For this review, use the dimensioned drawing (mm, ordinates from the lowest corner) and the shaded views. A direction names the side the tool comes from. Round coordinates to 2 decimals unless told otherwise and drop trailing zeros. Order: outer loops, then holes, each group sorted by start corner. A loop starts at its lowest first (then second) coordinate and runs counter-clockwise, first axis right, second up. Notation, with made-up numbers: M -34.5,48.25 L 16.5,48.25 A31 cw 16.5,84.25 Z; hole C -30,-18.5 d11. An arc over 180 degrees is marked long. One line per item, written item: value. Start each with the question number.
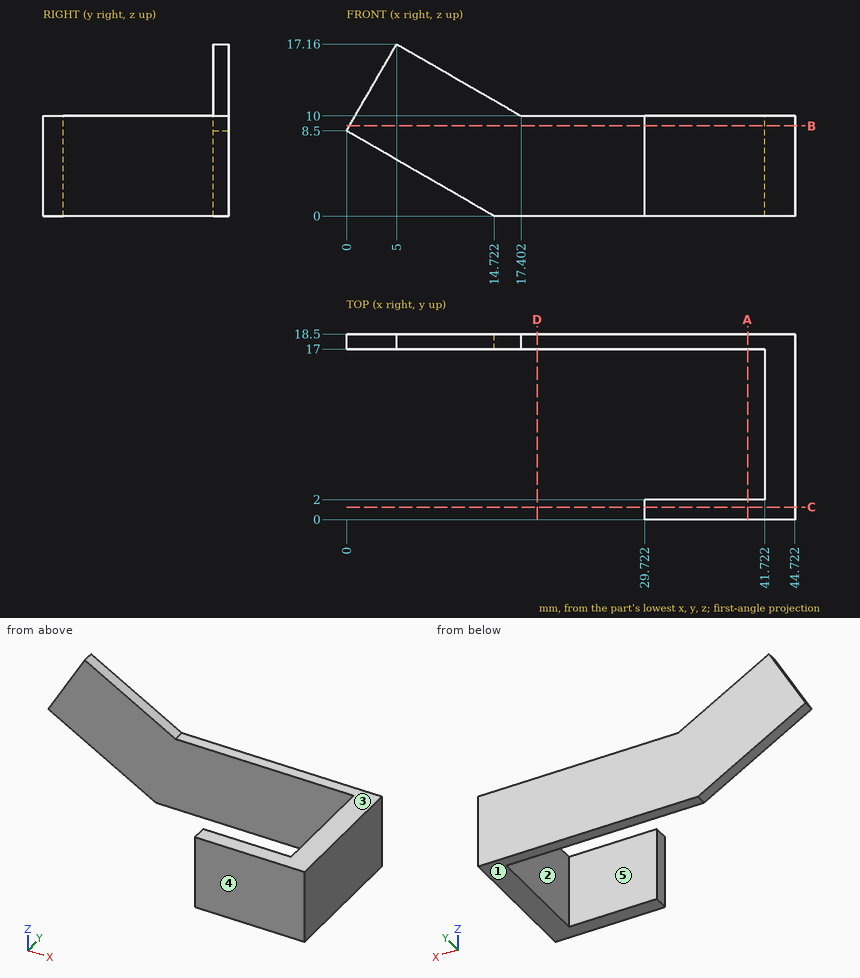
Item 1: Wall thickness on L1, parallel to X at y = 7.25, z = 8; L2, parallel to Y at x = 28.5, z = 6; L3, parallel to Y at x = 33.5, z = 6.25: over which ranges is each line inside the solid? List them lowest first.
Item 2: The part is to be moulded in two halves that separate along Y. For the marked faces 3, 4 and 5, say which applies: pulls with the +Y half, pulls with the -Y half, needs draft (parallel to the pull), parting line crosses it, or undercut.
Item 3: Consider section B-B, the plane z = 9. Give the boundary of the cut face in (x, y).
Item 4: Consider section D-D, the plane x = 19. Give the boundary of the cut face in (y, z).
Item 5: Consider section C-C, the plane y = 1.25. Give the boundary of the cut face in (x, z).
Item 6: Clearance check with flat-ended pins moving along their axes: P1, Ø6, axis at x = 40, y = 3, coming from the -Z side; P2, Ø10, axis at x = 17.5, z = 10.5, coming from the -Y side; P3, Ø1.6, axis at y = 1, z = 7.5, coming from the -X side; P4, Ø4, axis at y = 12.5, z = 13, coming from the -X side. State where each tip first meets the part, or that it passes through.
Item 7: Machinability: for the marked faces 1 and 2, which of the approach directions +Z, -Z, +X, -X, +Y, -Y give a long, thin tool a straight path to every point of the face, cutting with its end or side? Answer none if there is none.
Item 8: Consider section A-A, the plane x = 40. Give the boundary of the cut face in (y, z).
Computed:
1. L1: x = 41.72 to 44.72
1. L2: y = 17 to 18.5
1. L3: y = 0 to 2, 17 to 18.5
2. face 3: needs draft
2. face 4: pulls with the -Y half
2. face 5: undercut
3. outline: M 0.29,17 L 41.72,17 L 41.72,2 L 29.72,2 L 29.72,0 L 44.72,0 L 44.72,18.5 L 0.29,18.5 Z
4. outline: M 17,0 L 18.5,0 L 18.5,10 L 17,10 Z
5. outline: M 29.72,0 L 44.72,0 L 44.72,10 L 29.72,10 Z
6. P1: stops at z = 0
6. P2: stops at y = 17
6. P3: stops at x = 29.72
6. P4: passes through
7. face 1: -Z, +X, -X, +Y, -Y
7. face 2: +Z, -Z, -X
8. outline: M 0,0 L 2,0 L 2,10 L 0,10 Z; M 17,0 L 18.5,0 L 18.5,10 L 17,10 Z
